Verification items for the finished model (mm, model axes). Face numbers are marked on the shaded views. A direction names the side the tool comes from. Coordinates: 2 decimals unless noted, no trailing zeros. Write each loop counter-clockwise with the first axis right and the second up, starting at its lowest first coordinate (ties: lowest second). Pieces come first, ordered by that corner, then holes. Notation, with made-up numbers: (-20, 86) -> (30, 86) arc R34 ccw to (30, 123) -> close; hole circle Ø2 at (-39.5, -5). An arc over 180 degrees is marked (long way). Write item = value, one per line. Start each with the question number.
(1) Material ranges on probe 1 along Z at (x, y) = (12.7, 0.7); probe 2 along Z at (x, y) = (10.5, 2.25); probe 3 along X at (y, z) = (3.25, 3), recorded low to high. Write a range as [from, to].
(2) Mould release check, pull along X, two halves, no side actions. Record for the marked faces 5, 6 and 7: released by +X, released by -X, zero draft, split by the parting line, or undercut.
(3) Section check C-C (x = 11.5). Record the cut outline in (y, z).
(4) Gauge pin test, flat ends, axial feed: pin 1 Ø1.3 at (x, z) = (-7.5, 1) entering from -Y (3 decimals); pin 2 Ø1.5 at (x, z) = (14, -5) entering from +Y; pin 3 Ø3 at (x, z) = (15.5, 0) entering from +Y. Record the tip position at first contact, or that the pin passes through.
(5) Set-up check for the marked faces 1, 2, 3 and 4: record each of +Z, -Z, +X, -X, +Y, -Y from which the full face is reachable in a straight line by a thin tool's end or side.
(6) Section check B-B (y = 5.25). Record the cut outline in (x, z).
```python
from build123d import *

# Parameters (mm, degrees)
BOSS_EXTRUDE1_DEPTH            = 6.35
CUT_EXTRUDE3_START             = 1.5875
SKETCH4_W                      = 11.112499999999997
SKETCH4_H                      = 9.524999999999999
CUT_EXTRUDE3_DEPTH             = 24.057127330312788
CUT_EXTRUDE4_REACH             = 26.645
CUT_EXTRUDE4_DIRECTION_2_REACH = 26.645
SKETCH3_R                      = 2.5796875
CUT_EXTRUDE2_DEPTH             = 2.54


with BuildPart() as part:
    # Sketch1 → Boss-Extrude1 (new, symmetric)
    with BuildSketch(Plane.XY):
        with BuildLine():
            Line((-7.9375, 3.174999999999999), (-7.9375, 6.35))
            ThreePointArc((-7.9375, 6.35), (-3.487109685994719, 13.480495935616386), (4.873579631582188, 12.615151859662083))
            Line((4.873579631582188, 12.615151859662083), (19.049999999999997, 1.5875000000000004))
            Line((19.049999999999997, 1.5875000000000004), (19.049999999999997, 0))
            Line((19.049999999999997, 0), (6.350000000000001, -1.56e-15))
            Line((6.350000000000001, -1.56e-15), (6.35, 6.3500000000000005))
            ThreePointArc((6.35, 6.3500000000000005), (-1.02e-15, 12.7), (-6.35, 6.349999999999999))
            Line((-6.35, 6.349999999999999), (-6.35, 3.175))
            Line((-6.35, 3.175), (-7.9375, 3.174999999999999))
        make_face()
    extrude(amount=BOSS_EXTRUDE1_DEPTH, both=True)

    # Sketch4 → Cut-Extrude3 (cut, through all)
    with BuildSketch(Plane(origin=(0, 0, 0), x_dir=(1, 0, 0), z_dir=(0, 1, 0)).offset(CUT_EXTRUDE3_START)):
        with Locations((13.493749999999999, 0)):
            Rectangle(SKETCH4_W, SKETCH4_H)
    extrude(amount=CUT_EXTRUDE3_DEPTH, mode=Mode.SUBTRACT)

    # Cut-Extrude4: up to this face of the body (flat: up to its plane)
    cut_extrude4_end = Plane(part.part.faces().sort_by_distance((11.641666667, 4.468922769, 4.7625))[0])
    # Sketch5 → Cut-Extrude4 (cut, up to the picked face)
    with BuildSketch(Plane.XY, mode=Mode.PRIVATE) as cut_extrude4_sk1:
        with BuildLine():
            Line((7.9375, 6.35), (7.9375, 10.231768306511267))
            Line((7.9375, 10.231768306511267), (4.873579631582187, 12.615151859662081))
            ThreePointArc((4.873579631582187, 12.615151859662081), (7.130495935616386, 9.83710968599472), (7.9375, 6.35))
        make_face()
    cut_extrude4_tool1 = split(extrude(cut_extrude4_sk1.sketch, amount=CUT_EXTRUDE4_REACH, mode=Mode.PRIVATE), bisect_by=cut_extrude4_end, keep=Keep.BOTH, mode=Mode.PRIVATE)
    add(cut_extrude4_tool1.solids().sort_by(Axis((7.302263, 9.921111, 0), (0, 0, 1)))[0], mode=Mode.SUBTRACT)

    # Cut-Extrude4 direction 2: up to this face of the body (flat: up to its plane)
    cut_extrude4_direction_2_end = Plane(part.part.faces().sort_by_distance((11.641666667, 4.468922769, -4.7625))[0])
    # Sketch5 → Cut-Extrude4 direction 2 (cut, up to the picked face)
    with BuildSketch(Plane.XY, mode=Mode.PRIVATE) as cut_extrude4_direction_2_sk1:
        with BuildLine():
            Line((7.9375, 6.35), (7.9375, 10.231768306511267))
            Line((7.9375, 10.231768306511267), (4.873579631582187, 12.615151859662081))
            ThreePointArc((4.873579631582187, 12.615151859662081), (7.130495935616386, 9.83710968599472), (7.9375, 6.35))
        make_face()
    cut_extrude4_direction_2_tool1 = split(extrude(cut_extrude4_direction_2_sk1.sketch, amount=-CUT_EXTRUDE4_DIRECTION_2_REACH, mode=Mode.PRIVATE), bisect_by=cut_extrude4_direction_2_end, keep=Keep.BOTH, mode=Mode.PRIVATE)
    add(cut_extrude4_direction_2_tool1.solids().sort_by(Axis((7.302263, 9.921111, 0), (0, 0, -1)))[0], mode=Mode.SUBTRACT)

    # Sketch3 → Cut-Extrude2 (cut)
    with BuildSketch(Plane(origin=(0, 0, 0), x_dir=(1, 0, 0), z_dir=(0, 1, 0))):
        with Locations(Location((12.7, 0, 0), (0, 0, 270))):
            Circle(SKETCH3_R)
    extrude(amount=CUT_EXTRUDE2_DEPTH, mode=Mode.SUBTRACT)


solid = part.part
```
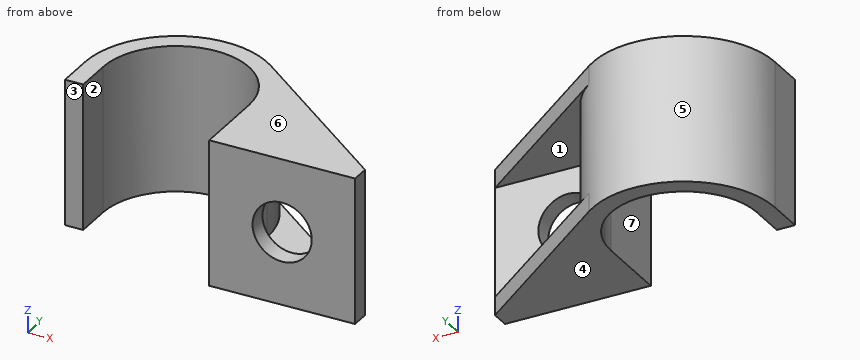
Response:
q1.probe_1 = [-6.35, -2.58], [2.58, 6.35]
q1.probe_2 = [-6.35, -4.76], [4.76, 6.35]
q1.probe_3 = [-7.94, -6.35], [6.35, 7.94]
q2.face_5 = split by the parting line
q2.face_6 = zero draft
q2.face_7 = undercut
q3.outline = (0, -6.35) -> (7.46, -6.35) -> (7.46, -4.76) -> (1.59, -4.76) -> (1.59, -2.28) -> (0, -2.28) -> close; (0, 2.28) -> (1.59, 2.28) -> (1.59, 4.76) -> (7.46, 4.76) -> (7.46, 6.35) -> (0, 6.35) -> close
q4.pin_1 = 3.175
q4.pin_2 = 6.1
q4.pin_3 = 1.59
q5.face_1 = +X, +Y
q5.face_2 = +Z, -Z, -Y
q5.face_3 = +Z, -Z, -X, -Y
q5.face_4 = -Z, +X, -X, +Y, -Y
q6.outline = (-7.94, -6.35) -> (-6.35, -6.35) -> (-6.35, 6.35) -> (-7.94, 6.35) -> close; (6.35, -6.35) -> (14.34, -6.35) -> (14.34, -4.76) -> (7.94, -4.76) -> (7.94, 4.76) -> (14.34, 4.76) -> (14.34, 6.35) -> (6.35, 6.35) -> close
